from build123d import *

# Parameters (mm, degrees)
SKETCH1_R           = 76.25
SKETCH1_R_2         = 69.75
BOSS_EXTRUDE1_DEPTH = 50.8
CHAMFER1_SIZE       = 2.5


with BuildPart() as part:
    # Sketch1 → Boss-Extrude1 (new body)
    with BuildSketch(Plane(origin=(0, 0, 0), x_dir=(1, 0, 0), z_dir=(0, 1, 0))):
        Circle(SKETCH1_R)
        Circle(SKETCH1_R_2, mode=Mode.SUBTRACT)
    extrude(amount=BOSS_EXTRUDE1_DEPTH)

    # Sketch2 → Cut-Revolve1 (revolve, cut)
    with BuildSketch(Plane.XY):
        Polygon((-76.25, 40.8), (-76.25, 36.55), (-73.75, 36.109182548), (-73.75, 41.240817452), align=None)
        Polygon((-73.75, 26.990817452), (-73.75, 21.859182548), (-76.25, 22.3), (-76.25, 26.55), align=None)
        Polygon((-73.75, 12.740817452), (-73.75, 7.609182548), (-76.25, 8.05), (-76.25, 12.3), align=None)
    revolve(axis=Axis((0, 0, 0), (0, 1, 0)), mode=Mode.SUBTRACT)

    # Chamfer1
    chamfer1_edges = [part.edges().sort_by_distance(p)[0] for p in [
        (-76.25, 0, 0),
    ]]
    chamfer(chamfer1_edges, length=CHAMFER1_SIZE)


solid = part.part
Design review of the part built by this model. Coordinates are the model's own, in mm. A direction names the side the tool comes from. Coordinates: 2 decimals unless noted, no trailing zeros. Write each loop counter-clockwise with the first axis right and the second up, starting at its lowest first coordinate (ties: lowest second). Pieces come first, ordered by that corner, then holes. Notation, with made-up numbers: (-4.5, 29.5) -> (19.5, 29.5) arc R14 ccw to (19.5, 39.5) -> close; hole circle Ø11 at (-10, 68). An arc over 180 degrees is marked (long way). Write each question's results on one line, items separated by ' | '. Start each with the question number.
(1) Clearance check with flat-ended pins moving along their axes: P1, Ø5, axis at x = -41.5, y = 24, coming from the -Z side; P2, Ø1, axis at y = 44, z = -39.5, coming from the -X side; P3, Ø1, axis at x = -8, y = 37.5, coming from the -Z side. State where each tip first meets the part, or that it passes through.
(2) For line 1 along X through (y, z) = (34.5, 0); line 2 along Y through (x, z) = (-24, -70), list the stretches that pass through material, from the lowest coordinate up. Write a range as from..to.
(3) Take a section at C-C on y = 19.5. Write out the cut boundary in (x, z).
(4) Tool access review of faces 4 (the face through (15.988, 24.389, -71.996)), 5 (the face through (-76.176, 17.23, -3.353)): name each direction out of +Z, -Z, +X, -X, +Y, -Y from which nothing blocks a thin tool from reaching the whole face with its end or side.
(5) The part is to be moulded in two halves that separate along Y. For faces 1 (the face through (58.65, 7.637, -44.971)), 2 (the face through (-76.176, 31.48, -3.353)), 3 (the face through (-16.014, 0.121, 72.115)), say which applies: pulls with the +Y half, pulls with the -Y half, needs draft (parallel to the pull), parting line crosses it, or undercut.
Results found:
1) P1: stops at z = -65.12 | P2: stops at x = -65.52 | P3: stops at z = -73.37
2) line 1: x = -76.25..-69.75, 69.75..76.25 | line 2: y = 0.25..7.65, 12.7..21.9, 26.95..36.15, 41.2..50.8
3) outline: circle Ø152.5 at (0, 0); hole circle Ø139.5 at (0, 0)
4) face 4: none | face 5: +Y, -Y
5) face 1: undercut | face 2: needs draft | face 3: pulls with the -Y half
